```python
from build123d import *

# Parameters (mm, degrees)
ESQUISSE1_W             = 113.4
ESQUISSE1_H             = 180
BOSS_EXTRU_1_DEPTH      = 3
ESQUISSE2_R             = 1.5
ENL_V_MAT_EXTRU_1_DEPTH = 10
ESQUISSE3_R             = 1.5
ENL_V_MAT_EXTRU_2_DEPTH = 10
ESQUISSE5_W             = 114.090437321
ESQUISSE5_H             = 45.152715072
ENL_V_MAT_EXTRU_3_DEPTH = 10
ENL_V_MAT_EXTRU_4_DEPTH = 10
CONG_2_R                = 8


with BuildPart() as part:
    # Esquisse1 → Boss.-Extru.1 (new body)
    with BuildSketch(Plane.XY):
        with Locations((56.7, 90)):
            Rectangle(ESQUISSE1_W, ESQUISSE1_H)
    extrude(amount=BOSS_EXTRU_1_DEPTH)

    # Esquisse2 → Enlèv. mat.-Extru.1 (cut)
    with BuildSketch(Plane.XY.offset(3)):
        with Locations((106.346648171, 50.037457394)):
            Circle(ESQUISSE2_R)
        with Locations((6.647370572, 50.037457394)):
            Circle(ESQUISSE2_R)
        with Locations((6.647370572, 125.962542606)):
            Circle(ESQUISSE2_R)
        with Locations((106.346648171, 125.962542606)):
            Circle(ESQUISSE2_R)
    extrude(amount=-ENL_V_MAT_EXTRU_1_DEPTH, mode=Mode.SUBTRACT)

    # Esquisse3 → Enlèv. mat.-Extru.2 (cut)
    with BuildSketch(Plane.XY.offset(3)):
        with Locations((76.706231896, 99.916374803)):
            Circle(ESQUISSE3_R)
        with Locations((36.706231896, 99.916374803)):
            Circle(ESQUISSE3_R)
        with Locations((84.706231896, 169.916374803)):
            Circle(ESQUISSE3_R)
        with Locations((28.675912775, 169.916374803)):
            Circle(ESQUISSE3_R)
    extrude(amount=-ENL_V_MAT_EXTRU_2_DEPTH, mode=Mode.SUBTRACT)

    # Esquisse5 → Enlèv. mat.-Extru.3 (cut)
    with BuildSketch(Plane.XY.offset(3)):
        with Locations((56.35478134, 21.269970053)):
            Rectangle(ESQUISSE5_W, ESQUISSE5_H)
    extrude(amount=-ENL_V_MAT_EXTRU_3_DEPTH, mode=Mode.SUBTRACT)

    # Esquisse6 → Enlèv. mat.-Extru.4 (cut)
    with BuildSketch(Plane.XY.offset(3)):
        with BuildLine():
            Line((99.394396977, 43.846327589), (13.780181086, 43.846327589))
            ThreePointArc((13.780181086, 43.846327589), (56.587289031, 74.506937859), (99.394396977, 43.846327589))
        make_face()
    extrude(amount=-ENL_V_MAT_EXTRU_4_DEPTH, mode=Mode.SUBTRACT)

    # Congé2
    cong_2_edges = [part.edges().sort_by_distance(p)[0] for p in [
        (99.394396977, 43.846327589, 1.5),
        (13.780181086, 43.846327589, 1.5),
    ]]
    fillet(cong_2_edges, radius=CONG_2_R)


solid = part.part
```
Can you work these out from the model? Positions are in its coordinate system, mm. A direction names the side the tool comes from. Give positions to 0.01 mm unless a question says otherwise; leave off trailing zeros. Loops run counter-clockwise (first coordinate to the right, second up) from the corner with the lowest first, then second, coordinate; pieces in that order, holes last. Notation, with made-up numbers: M 56,7.5 L 85,7.5 A15 cw 85,22.5 Z; hole C 9,42 d1. An arc over 180 degrees is marked long. Use CSV: the item, a comma, the result in double quotes. Start each with the question number.
1. Imagine slicing it at B-B, the plane z = 1.8. Count the separate pieces of the cut face and the enclosed holes in it, plus the area to 3 significant figures.
2. If we mould it in two halves opening along X, with no side actions, what happens to faces 1 (the face through (56, 128, 3)), 2 (the face through (28.481, 171.404, 1.521)), 3 (the face through (0, 111, 1))? For each: released by +X, released by -X, zero draft, split by the parting line, or undercut.
3. Imagine slicing it at C-C, the plane x = 21.5. Write out the boundary of the cut face in (y, z).
4. For P1, Ø1.8, axis at x = 106.35, y = 125.96, coming from the +Z side; P2, Ø3.5, axis at x = 6.65, y = 125.96, coming from the -Z side, each with a flat end and sliding along its axis, tell me the tip position at first contact or that it passes through.
5. If I drill on L1, parallel to X at y = 55, z = 1.65; L2, parallel to X at y = 59, z = 2.45; L3, parallel to Y at x = 37, z = 1.05, over which ranges is the centre line in solid material (lowest first)?
6. On a 3-axis mill with a long thin cutter (end or side, diameter ignored), from which of +Z, -Z, +X, -X, +Y, -Y can I reach the whole of each face in a straight line? I mean faces 4 (the face through (113.4, 111, 1)), 5 (the face through (12.63, 45.063, 1.479)). Say none if no direction works.
7. Imagine slicing it at A-A, the plane y = 56.5. Write out the boundary of the cut face in (x, z), plus the area to 3 significant figures.
Response values:
1,separate pieces,"1"
1,enclosed holes,"8"
1,area,"13,500 mm^2"
2,face 1,"zero draft"
2,face 2,"undercut"
2,face 3,"released by -X"
3,outline,"M 57.81,0 L 180,0 L 180,3 L 57.81,3 Z"
4,P1,"through"
4,P2,"z = 0"
5,L1,"0 to 19.39, 93.78 to 113.4"
5,L2,"0 to 22.5, 90.67 to 113.4"
5,L3,"70.04 to 98.45, 101.39 to 180"
6,face 4,"+Z, -Z, +X, +Y, -Y"
6,face 5,"+Z, -Z, -Y"
7,outline,"M 0,0 L 20.48,0 L 20.48,3 L 0,3 Z; M 92.7,0 L 113.4,0 L 113.4,3 L 92.7,3 Z"
7,area,"124 mm^2"
